from build123d import *

# Parameters (mm, degrees)
CHAMFER_1_SIZE = 0.5


with BuildPart() as part:
    # Sketch 1 → Revolve 1 (revolve)
    with BuildSketch(Plane.XY):
        Polygon((59.45, 0), (59.45, 5), (58.25, 5), (58.25, 4.8), (57.15, 4.8), (57.15, 5), (-57.15, 5), (-57.15, 4.8), (-58.25, 4.8), (-58.25, 5), (-59.45, 5), (-59.45, 0), align=None)
    revolve(axis=Axis((59.45, 0, 0), (-1, 0, 0)))

    # Chamfer 1
    chamfer_1_edges = [part.edges().sort_by_distance(p)[0] for p in [
        (-59.45, -5, 0),
        (59.45, -5, 0),
    ]]
    chamfer(chamfer_1_edges, length=CHAMFER_1_SIZE)


solid = part.part
Model file for the job. Use its own axes, mm. A direction names the side the tool comes from. Give positions to 0.01 mm unless a question says otherwise; leave off trailing zeros. Put each result on its own line as item: value. Start each with the question number.
(1) Tool access for faces 4 (the face through (57.69, 2.58, -4.05)), 5 (the face through (-58.6, -1.08, 4.88)): list every direction of +Z, -Z, +X, -X, +Y, -Y with a clear straight run to the whole face (end or side of a thin tool).
(2) Pin check, flat tips, straight feed: pin 1 Ø1.5 at (x, y) = (-44, 1) entering from -Z; pin 2 Ø1.5 at (x, z) = (-20.5, -3) entering from -Y; pin 3 Ø1.5 at (x, z) = (-18, -1.5) entering from +Y. Stop position of each tip, or through.
(3) Pull direction X, two halves, no side cores. Call faces 1 (the face through (-57.71, 2.58, -4.05)), 2 (the face through (-0.8, -1.08, 4.88)), 3 (the face through (59.45, 0, 0)): released by +X, released by -X, zero draft, split by the parting line, or undercut.
(4) Drill centre lines: L1, parallel to X at y = 3.75, z = 2.5; L2, parallel to Z at x = 5.5, y = -0.25; L3, parallel to Y at x = -32.5, z = -4. Where is each one in solid material? Low to high. Write a range as [from, to].
Results below:
1. face 4: none
1. face 5: +X, -X
2. pin 1: stops at z = -4.99
2. pin 2: stops at y = -4.47
2. pin 3: stops at y = 4.94
3. face 1: undercut
3. face 2: zero draft
3. face 3: released by +X
4. L1: x = [-59.44, 59.44]
4. L2: z = [-4.99, 4.99]
4. L3: y = [-3, 3]
